Model file for the job. Use its own axes, mm. A direction names the side the tool comes from. Round coordinates to 2 decimals unless told otherwise and drop trailing zeros. Order: outer loops, then holes, each group sorted by start corner. A loop starts at its lowest first (then second) coordinate and runs counter-clockwise, first axis right, second up. Notation, with made-up numbers: (71, -7.5) - (107, -7.5) arc R19 cw to (107, 18.5) - close; hole circle Ø10 at (-28, 45). An arc over 180 degrees is marked (long way). Put each result on its own line as item: value. Start each with the question number.
Item 1: Saw through at B-B on y = -6. List the corners of the cut face in (x, z), plus the area to 3 significant figures.
Item 2: Saw through at A-A on y = -16. List the corners of the cut face in (x, z), plus the area to 3 significant figures.
Item 3: Probe probe 1 along Y at (x, z) = (27.7, 0); probe 2 along Y at (x, z) = (-25.45, 0); probe 3 along X at (y, z) = (-37, 13.5). List the from-to ranges inside material, lowest first.
Item 4: Which spindle directions (+Z, -Z, +X, -X, +Y, -Y) get a long thin tool onto all of the face, cutting with end or side? Do faces 1 (the face through (-18.633, -40.523, -10.224)), 2 (the face through (0, -34, -32)), 3 (the face through (28.4, -10.53, -15.4)). Say none if no direction does.
Item 5: Pin check, flat tips, straight feed: pin 1 Ø22 at (y, z) = (-29, -1.5) entering from -X; pin 2 Ø1 at (x, y) = (-21.5, -36.5) entering from -Z; pin 3 Ø12 at (x, z) = (9, -24) entering from -Y. Stop position of each tip, or through.
Item 6: Mould opens along Y. For faces 4 (the face through (-27.507, -23.077, 1.172)), 5 (the face through (-22.92, -43.78, 24.33)), 6 (the face through (-19, -24, 12)) say: pulls with the +Y half, pulls with the -Y half, needs draft (parallel to the pull), parting line crosses it, or undercut.
```python
from build123d import *

# Parameters (mm, degrees)
BOSS_EXTRUDE1_REACH     = 68.895
CUT_EXTRUDE1_DEPTH      = 67.895440801
CUT_EXTRUDE1_DEPTH_BACK = 26
CUT_EXTRUDE5_START      = -56
CUT_EXTRUDE5_OUTLINE_R  = 9
CUT_EXTRUDE5_DEPTH      = 56
CUT_EXTRUDE6_START      = -1
SKETCH5_R               = 10
CUT_EXTRUDE6_DEPTH      = 2


# Read off the part's stored shape, not the designer's step: Cut-Extrude5
with BuildPart() as part:
    # Sketch1 → Revolve6 (revolve)
    with BuildSketch(Plane.XY, mode=Mode.PRIVATE) as revolve6_sk:
        Polygon((0, 0), (34.5, 0), (35, -0.5), (35, -3.530079997), (32, -3.530079997), (32, -5.030079997), (35, -5.030079997), (35, -7.030079997), (32, -7.030079997), (32, -8.530079997), (35, -8.530079997), (35, -10.530079997), (32, -10.530079997), (32, -14.530079997), (35, -14.530079997), (35, -45), (32, -45), (32, -23.460781634), (25, -17), (25, -7), (0, -7), align=None)
    revolve(revolve6_sk.sketch.rotate(Axis((0, -7, 0), (0, 1, 0)), 90), axis=Axis((0, -7, 0), (0, 1, 0)))

    # Sketch2 → Boss-Extrude1 (add, up to next)
    with BuildSketch(Plane.XZ.offset(45), mode=Mode.PRIVATE) as boss_extrude1_sk1:
        with BuildLine():
            Line((-25, 19.974984355), (-25, 12))
            Line((-25, 12), (-12, 12))
            ThreePointArc((-12, 12), (-9.878679656, 11.121320344), (-9, 9))
            Line((-9, 9), (-9, -9))
            ThreePointArc((-9, -9), (-9.878679656, -11.121320344), (-12, -12))
            Line((-12, -12), (-25, -12))
            Line((-25, -12), (-25, -19.974984355))
            ThreePointArc((-25, -19.974984355), (-32, 0), (-25, 19.974984355))
        make_face()
    boss_extrude1_tool1 = extrude(boss_extrude1_sk1.sketch, amount=-BOSS_EXTRUDE1_REACH, mode=Mode.PRIVATE) - part.part
    # Sketch2 → Boss-Extrude1 (add, up to next)
    with BuildSketch(Plane.XZ.offset(45), mode=Mode.PRIVATE) as boss_extrude1_sk2:
        with BuildLine():
            Line((25, 19.974984355), (25, 12))
            Line((25, 12), (12, 12))
            ThreePointArc((12, 12), (9.878679656, 11.121320344), (9, 9))
            Line((9, 9), (9, -9))
            ThreePointArc((9, -9), (9.878679656, -11.121320344), (12, -12))
            Line((12, -12), (25, -12))
            Line((25, -12), (25, -19.974984355))
            ThreePointArc((25, -19.974984355), (32, 0), (25, 19.974984355))
        make_face()
    boss_extrude1_tool2 = extrude(boss_extrude1_sk2.sketch, amount=-BOSS_EXTRUDE1_REACH, mode=Mode.PRIVATE) - part.part
    add(boss_extrude1_tool1.solids().sort_by_distance((-20.669877, -45, 0))[0])
    add(boss_extrude1_tool2.solids().sort_by_distance((20.669877, -45, 0))[0])

    # Sketch3 → Cut-Extrude1 (cut, two sides: drawn at the far end of the back side and taken through both)
    with BuildSketch(Plane.XZ.offset(45).offset(-CUT_EXTRUDE1_DEPTH_BACK)):
        with BuildLine():
            Line((-28, 21), (-28, -21))
            ThreePointArc((-28, -21), (-35, 0), (-28, 21))
        make_face()
        with BuildLine():
            Line((28, 21), (28, -21))
            ThreePointArc((28, -21), (35, 0), (28, 21))
        make_face()
    extrude(amount=CUT_EXTRUDE1_DEPTH + CUT_EXTRUDE1_DEPTH_BACK, mode=Mode.SUBTRACT)

    # Cut-Extrude5 outline → Cut-Extrude5 (cut)
    with BuildSketch(Plane(origin=(28, 0, 0), x_dir=(0, 0, -1), z_dir=(1, 0, 0)).offset(CUT_EXTRUDE5_START)):
        with BuildLine():
            Line((19.292173786, -40), (12.449899598, -40))
            ThreePointArc((12.449899598, -40), (10.586509617, -40.360196364), (8.991594154, -41.388888889))
            ThreePointArc((8.991594154, -41.388888889), (4.84481396, -44.063489449), (1.9e-08, -45))
            Line((1.9e-08, -45), (25, -45))
            Line((25, -45), (23.672124938, -42.588355767))
            ThreePointArc((23.672124938, -42.588355767), (21.835968082, -40.69545466), (19.292173786, -40))
        make_face()
        with BuildLine():
            ThreePointArc((1.9e-08, -45), (-4.844813942, -44.063489456), (-8.991594154, -41.388888889))
            ThreePointArc((-8.991594154, -41.388888889), (-10.586509617, -40.360196364), (-12.449899598, -40))
            Line((-12.449899598, -40), (-19.292173786, -40))
            ThreePointArc((-19.292173786, -40), (-21.835968082, -40.69545466), (-23.672124938, -42.588355767))
            Line((-23.672124938, -42.588355767), (-25, -45))
            Line((-25, -45), (1.9e-08, -45))
        make_face()
        with Locations((0, -32)):
            Circle(CUT_EXTRUDE5_OUTLINE_R)
    extrude(amount=CUT_EXTRUDE5_DEPTH, mode=Mode.SUBTRACT)

    # Sketch5 → Cut-Extrude6 (cut)
    with BuildSketch(Plane(origin=(28, 0, 0), x_dir=(0, 0, -1), z_dir=(1, 0, 0)).offset(CUT_EXTRUDE6_START)):
        with Locations((0, -32)):
            Circle(SKETCH5_R)
    cut_extrude6 = extrude(amount=-CUT_EXTRUDE6_DEPTH, mode=Mode.SUBTRACT)

    # Mirror1: Cut-Extrude6 across plane
    add(cut_extrude6.mirror(Plane(origin=(0, 0, 0), x_dir=(0, 0, 1), z_dir=(1, 0, 0))), mode=Mode.SUBTRACT)


solid = part.part
```
Results found:
1. outline: circle Ø70 at (0, 0)
1. area: 3,850 mm²
2. outline: circle Ø70 at (0, 0); hole (-21.93, -12) arc R25 ccw to (21.93, -12) - (12, -12) arc R3 cw to (9, -9) - (9, 9) arc R3 cw to (12, 12) - (21.93, 12) arc R25 ccw to (-21.93, 12) - (-12, 12) arc R3 cw to (-9, 9) - (-9, -9) arc R3 cw to (-12, -12) - close
2. area: 2,600 mm²
3. probe 1: y = -45 to -41, -23 to 0
3. probe 2: y = -45 to -42, -22 to 0
3. probe 3: x = -28 to -25, 25 to 28
4. face 1: +X, -X, -Y
4. face 2: -Y
4. face 3: none
5. pin 1: stops at x = -35
5. pin 2: stops at z = -28
5. pin 3: stops at y = -23.12
6. face 4: undercut
6. face 5: pulls with the -Y half
6. face 6: needs draft
